Can you work these out from the model? Positions are in its coordinate system, mm. A direction names the side the tool comes from. Coordinates: 2 decimals unless noted, no trailing zeros. Order: outer loops, then holes, each group sorted by start corner. A loop starts at its lowest first (then second) coordinate and runs counter-clockwise, first axis right, second up. Notation, with made-up numbers: (-32.5, -19) -> (6.5, -19) arc R14 cw to (6.5, 0) -> close; hole circle Ø4 at (75.25, 14.25). An arc over 180 degrees is marked (long way). Write item = value, one per line. Start each with the question number.
from build123d import *

# Parameters (mm, degrees)
F0_R     = 14.5415
F1_DEPTH = 10.16
F4_DEPTH = 25.4
F5_DEPTH = 25.4
F6_R     = 5.715
F7_DEPTH = 25.4
F8_W     = 25.4
F8_H     = 11.43
F9_DEPTH = 19.05


with BuildPart() as f1:
    # F0 (on Front) → F1 (new body)
    with BuildSketch(Plane.XZ):
        Circle(F0_R)
    extrude(amount=F1_DEPTH)

    # F3 (on Right) → F4 (join)
    with BuildSketch(Plane.YZ):
        Polygon((-10.16, -14.225606), (0.017161, -14.225606), (-10.16, 0.135286), align=None)
    extrude(amount=F4_DEPTH)

    # F2 (on Right) → F5 (join)
    with BuildSketch(Plane.YZ):
        Polygon((-0.017161, 14.5415), (-10.194321, 14.5415), (-0.017161, 0.180608), align=None)
    extrude(amount=-F5_DEPTH)

    # F6 (on Front) → F7 (join)
    with BuildSketch(Plane.XZ):
        Circle(F6_R)
    extrude(amount=-F7_DEPTH)

    # F8 (on face) → F9 (join)
    with BuildSketch(Plane(origin=(0, 25.4, 0), x_dir=(-1, 0, 0), z_dir=(0, 1, 0))):
        Rectangle(F8_W, F8_H)
    extrude(amount=F9_DEPTH)


solid = f1.part
(1) For faces 5 (the face through (0, 35, 5.715)), 6 (the face through (0, 35, -5.715)), 7 (the face through (6, 0, 0)), 8 (the face through (12.7, 35, 0)), which set-ups out of +Z, -Z, +X, -X, +Y, -Y let a thin tool reach every point of the face, with its end or its side?
(2) For P1, Ø10, axis at x = 5.5, y = 28.5, coming from the +Z side (3 decimals); P2, Ø3, axis at x = 2, z = -7, coming from the -Y side; P3, Ø4, axis at x = -9, y = 26, coming from the -Z side (3 decimals); P4, Ø10, axis at y = 19, z = -11, coming from the +X side, each with a flat end and sliding along its axis, tell me the tip position at first contact or that it passes through.
(3) If I drill on L1, parallel to Y at x = 12, z = 0; L2, parallel to Y at x = 13.5, z = -4.25; L3, parallel to Z at x = 0, y = 28.5 (3 decimals), over which ranges is the centre line in solid material (lowest first)? Write a range as from..to.
(4) Imagine slicing it at B-B (y = -2). Write out the boundary of the cut face in (x, z).
(5) Imagine slicing it at D-D (x = 19). Write out the boundary of the cut face in (y, z).
(6) Thinking about a two-plate mould opening in Z: for faces 1 (the face through (25.4, -7, -10)), 2 (the face through (-18.167, -5.177, 7.462)), 3 (the face through (18.167, -5, -7.146)), 4 (the face through (-13, -5, 14.542)), which applies, +Z half, -Z half, draft (parallel to the pull), parting line (faces both ways), or undercut?
(7) Imagine slicing it at A-A (x = 9). Write out the boundary of the cut face in (y, z) (3 decimals).
Result set:
q1.face_5 = +Z, +X, -X, +Y
q1.face_6 = -Z, +X, -X, +Y
q1.face_7 = none
q1.face_8 = +Z, -Z, +X, +Y
q2.P1 = 5.715
q2.P2 = -10.16
q2.P3 = -5.715
q2.P4 = through
q3.L1 = -10.16..0, 25.4..44.45
q3.L2 = -10.16..0
q3.L3 = -5.715..5.715
q4.outline = (-25.4, 2.98) -> (-14.23, 2.98) arc R14.54 ccw to (3.01, -14.23) -> (25.4, -14.23) -> (25.4, -11.38) -> (9.05, -11.38) arc R14.54 ccw to (0, 14.54) -> (-25.4, 14.54) -> close
q5.outline = (-10.16, -14.23) -> (0.02, -14.23) -> (-10.16, 0.14) -> close
q6.face_1 = draft
q6.face_2 = undercut
q6.face_3 = undercut
q6.face_4 = +Z half
q7.outline = (-10.16, -14.226) -> (0.017, -14.226) -> (-1.97, -11.422) -> (0, -11.422) -> (0, 11.422) -> (-10.16, 11.422) -> close; (25.4, -5.715) -> (44.45, -5.715) -> (44.45, 5.715) -> (25.4, 5.715) -> close
